Work out the finished part from the listing and answer in its coordinate system (mm). Face numbers are marked on the shaded views. A direction names the side the tool comes from. Round coordinates to 2 decimals unless told otherwise and drop trailing zeros. Order: outer loops, then holes, each group sorted by start corner. A loop starts at its lowest first (then second) coordinate and runs counter-clockwise, first axis right, second up. Notation, with made-up numbers: (-3, 67.5) - (52, 67.5) arc R26 cw to (52, 106.5) - close; hole circle Ø5 at (-19, 2). An arc over 180 degrees is marked (long way). Answer in a Markdown table with one row per item.
from build123d import *

# Parameters (mm, degrees)
ESQUISSE2_W           = 165
ESQUISSE2_H           = 165
BASE_DEPTH            = 30
ESQUISSE3_R           = 15
BLOC_MOTEUR_1_DEPTH   = 80
ESQUISSE4_W           = 10
ESQUISSE4_H           = 22.360679774
ACCES_MOTEUR_DEPTH    = 37
ESQUISSE6_R           = 16.01
BLOC_MOTEUR_2_DEPTH   = 37
ESQUISSE7_R           = 2.5
VIS_MOTEUR_DEPTH      = 121.467838032
ESQUISSE8_R           = 2.5
VIS_PATIN_DEPTH       = 121.467838032
ESQUISSE9_R           = 3.1
ESQUISSE9_R_2         = 1.375
SUPPORT_RASP_DEPTH    = 10
ESQUISSE11_R          = 2.5
ESQUISSE11_R_2        = 1.6
SUPPORT_ARDUINO_DEPTH = 10
CONGE_EXT_R           = 5
ESQUISSE12_R          = 30
ESPACE_ROUE_DEPTH     = 10


with BuildPart() as part:
    # Esquisse2 → BASE (new body)
    with BuildSketch(Plane(origin=(0, 0, 0), x_dir=(1, 0, 0), z_dir=(0, 1, 0))):
        Rectangle(ESQUISSE2_W, ESQUISSE2_H)
    extrude(amount=BASE_DEPTH)

    # Esquisse3 → BLOC MOTEUR 1. (cut)
    with BuildSketch(Plane(origin=(82.5, 0, 0), x_dir=(0, 0, -1), z_dir=(1, 0, 0))):
        with Locations((50, 10)):
            Circle(ESQUISSE3_R)
    bloc_moteur_1 = extrude(amount=-BLOC_MOTEUR_1_DEPTH, mode=Mode.SUBTRACT)

    # Esquisse4 → ACCES MOTEUR (cut)
    with BuildSketch(Plane.XZ):
        with Locations((7.5, -50)):
            Rectangle(ESQUISSE4_W, ESQUISSE4_H)
    acces_moteur = extrude(amount=-ACCES_MOTEUR_DEPTH, mode=Mode.SUBTRACT)

    # Esquisse6 → BLOC MOTEUR 2 (cut)
    with BuildSketch(Plane(origin=(82.5, 0, 0), x_dir=(0, 0, -1), z_dir=(1, 0, 0))):
        with Locations((50, 10)):
            Circle(ESQUISSE6_R)
    bloc_moteur_2 = extrude(amount=-BLOC_MOTEUR_2_DEPTH, mode=Mode.SUBTRACT)

    # SYM BLOC MOTEUR: BLOC MOTEUR 1., ACCES MOTEUR, BLOC MOTEUR 2 across plane
    add(bloc_moteur_1.mirror(Plane(origin=(0, 0, 0), x_dir=(0, 0, 1), z_dir=(1, 0, 0))), mode=Mode.SUBTRACT)
    add(acces_moteur.mirror(Plane(origin=(0, 0, 0), x_dir=(0, 0, 1), z_dir=(1, 0, 0))), mode=Mode.SUBTRACT)
    add(bloc_moteur_2.mirror(Plane(origin=(0, 0, 0), x_dir=(0, 0, 1), z_dir=(1, 0, 0))), mode=Mode.SUBTRACT)

    # Esquisse7 → VIS MOTEUR (cut, through all)
    with BuildSketch(Plane.XZ):
        with Locations(Location((-64, -27.497196314, 0), (0, 0, 270))):
            Circle(ESQUISSE7_R)
        with Locations(Location((-24, -28.819660113, 0), (0, 0, 270))):
            Circle(ESQUISSE7_R)
        with Locations(Location((-24, -71.180339887, 0), (0, 0, 270))):
            Circle(ESQUISSE7_R)
        with Locations(Location((-64, -72.502803686, 0), (0, 0, 270))):
            Circle(ESQUISSE7_R)
    vis_moteur = extrude(amount=-VIS_MOTEUR_DEPTH, mode=Mode.SUBTRACT)

    # SYM VIS: VIS MOTEUR across plane
    add(vis_moteur.mirror(Plane(origin=(0, 0, 0), x_dir=(0, 0, 1), z_dir=(1, 0, 0))), mode=Mode.SUBTRACT)

    # Esquisse8 → VIS PATIN (cut, through all)
    with BuildSketch(Plane.XZ):
        with Locations(Location((-52.5, 52.5, 0), (0, 0, 270))):
            Circle(ESQUISSE8_R)
        with Locations(Location((52.5, 52.5, 0), (0, 0, 270))):
            Circle(ESQUISSE8_R)
    extrude(amount=-VIS_PATIN_DEPTH, mode=Mode.SUBTRACT)

    # Esquisse9 → SUPPORT RASP (add)
    # profile 1 of 4: a face of its own
    with BuildSketch(Plane(origin=(0, 30, 0), x_dir=(1, 0, 0), z_dir=(0, 1, 0))):
        with Locations(Location((-5.124679211, -22.194338496, 0), (0, 0, 90))):
            Circle(ESQUISSE9_R)
        with Locations(Location((-5.124679211, -22.194338496, 0), (0, 0, 270))):
            Circle(ESQUISSE9_R_2, mode=Mode.SUBTRACT)
    # profile 2 of 4: a face of its own
    with BuildSketch(Plane(origin=(0, 30, 0), x_dir=(1, 0, 0), z_dir=(0, 1, 0))):
        with Locations(Location((52.875320789, -22.194338496, 0), (0, 0, 90))):
            Circle(ESQUISSE9_R)
        with Locations(Location((52.875320789, -22.194338496, 0), (0, 0, 270))):
            Circle(ESQUISSE9_R_2, mode=Mode.SUBTRACT)
    # profile 3 of 4: a face of its own
    with BuildSketch(Plane(origin=(0, 30, 0), x_dir=(1, 0, 0), z_dir=(0, 1, 0))):
        with Locations(Location((-5.124679211, -71.194338496, 0), (0, 0, 90))):
            Circle(ESQUISSE9_R)
        with Locations(Location((-5.124679211, -71.194338496, 0), (0, 0, 270))):
            Circle(ESQUISSE9_R_2, mode=Mode.SUBTRACT)
    # profile 4 of 4: a face of its own
    with BuildSketch(Plane(origin=(0, 30, 0), x_dir=(1, 0, 0), z_dir=(0, 1, 0))):
        with Locations(Location((52.875320789, -71.194338496, 0), (0, 0, 90))):
            Circle(ESQUISSE9_R)
        with Locations(Location((52.875320789, -71.194338496, 0), (0, 0, 270))):
            Circle(ESQUISSE9_R_2, mode=Mode.SUBTRACT)
    extrude(amount=SUPPORT_RASP_DEPTH)

    # Esquisse11 → SUPPORT ARDUINO (add)
    # profile 1 of 4: a face of its own
    with BuildSketch(Plane(origin=(0, 30, 0), x_dir=(1, 0, 0), z_dir=(0, 1, 0))):
        with Locations(Location((-70.933772323, -17.670594659, 0), (0, 0, 90))):
            Circle(ESQUISSE11_R)
        with Locations(Location((-70.933772323, -17.670594659, 0), (0, 0, 270))):
            Circle(ESQUISSE11_R_2, mode=Mode.SUBTRACT)
    # profile 2 of 4: a face of its own
    with BuildSketch(Plane(origin=(0, 30, 0), x_dir=(1, 0, 0), z_dir=(0, 1, 0))):
        with Locations(Location((-23.123772323, -18.770594659, 0), (0, 0, 90))):
            Circle(ESQUISSE11_R)
        with Locations(Location((-23.123772323, -18.770594659, 0), (0, 0, 270))):
            Circle(ESQUISSE11_R_2, mode=Mode.SUBTRACT)
    # profile 3 of 4: a face of its own
    with BuildSketch(Plane(origin=(0, 30, 0), x_dir=(1, 0, 0), z_dir=(0, 1, 0))):
        with Locations(Location((-66.233772323, -60.010594659, 0), (0, 0, 90))):
            Circle(ESQUISSE11_R)
        with Locations(Location((-66.233772323, -60.010594659, 0), (0, 0, 270))):
            Circle(ESQUISSE11_R_2, mode=Mode.SUBTRACT)
    # profile 4 of 4: a face of its own
    with BuildSketch(Plane(origin=(0, 30, 0), x_dir=(1, 0, 0), z_dir=(0, 1, 0))):
        with Locations(Location((-38.333772323, -60.010594659, 0), (0, 0, 90))):
            Circle(ESQUISSE11_R)
        with Locations(Location((-38.333772323, -60.010594659, 0), (0, 0, 270))):
            Circle(ESQUISSE11_R_2, mode=Mode.SUBTRACT)
    extrude(amount=SUPPORT_ARDUINO_DEPTH)

    # CONGE EXT
    conge_ext_edges = [part.edges().sort_by_distance(p)[0] for p in [
        (-82.5, 15, -82.5),
        (82.5, 15, -82.5),
        (82.5, 15, 82.5),
        (-82.5, 15, 82.5),
    ]]
    fillet(conge_ext_edges, radius=CONGE_EXT_R)

    # Esquisse12 → ESPACE ROUE (cut)
    with BuildSketch(Plane.ZY.offset(82.5)):
        with Locations((-50, 10)):
            Circle(ESQUISSE12_R)
    espace_roue = extrude(amount=-ESPACE_ROUE_DEPTH, mode=Mode.SUBTRACT)

    # SYM ESPACE ROUE: ESPACE ROUE across plane
    add(espace_roue.mirror(Plane(origin=(0, 0, 0), x_dir=(0, 0, 1), z_dir=(1, 0, 0))), mode=Mode.SUBTRACT)


solid = part.part
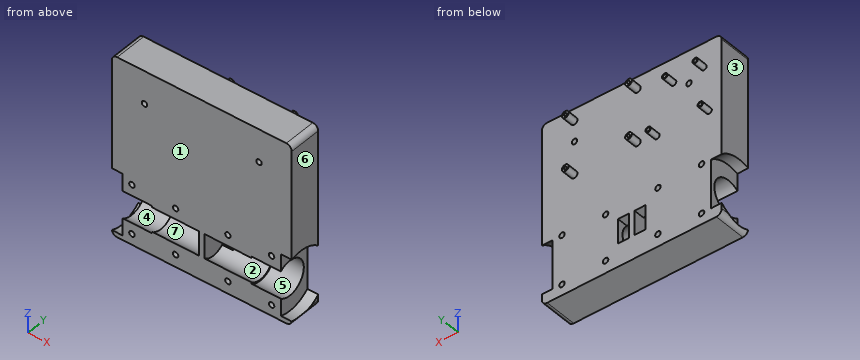
1) Find section B-B, the plane x = 24. Give the vertices of the cut face in (y, z), then the cut area to 3 significant figures.
Filled in:
| item | result |
|---|---|
| outline | (0, -82.5) - (30, -82.5) - (30, -73.68) - (0, -73.68) - close; (0, -68.68) - (30, -68.68) - (30, -31.32) - (0, -31.32) - (0, -38.82) arc R15 cw (long way) to (0, -61.18) - close; (0, -26.32) - (30, -26.32) - (30, 82.5) - (0, 82.5) - close |
| area | 4,020 mm^2 |
2) Find section D-D, the plane y = 16. Give the number of separate pieces and of enclosed holes in the cut face, then the cut area to 3 significant figures.
Filled in:
| item | result |
|---|---|
| separate pieces | 1 |
| enclosed holes | 10 |
| area | 21,900 mm^2 |
3) Find section C-C, the plane x = -52.5. Give the vertices of the cut face in (y, z).
Filled in:
| item | result |
|---|---|
| outline | (0, -82.5) - (30, -82.5) - (30, 50) - (0, 50) - (0, -37.5) arc R16.01 cw (long way) to (0, -62.5) - close; (0, 55) - (30, 55) - (30, 82.5) - (0, 82.5) - close |
4) Find section A-A, the plane z = 52.5. Give the vertices of the cut face in (x, y).
Filled in:
| item | result |
|---|---|
| outline | (-82.5, 0) - (-55, 0) - (-55, 30) - (-82.5, 30) - close; (-50, 0) - (50, 0) - (50, 30) - (-50, 30) - close; (55, 0) - (82.5, 0) - (82.5, 30) - (55, 30) - close |
5) Each of these flat-tipped pins is pushed along its axis until it touches: pin 1 (1.5 mm diameter, centred on y = 31, z = 42.5, fed in from +X); pin 2 (1.6 mm diameter, centred on x = -66.5, z = 60.5, fed in from +Y); pin 3 (24 mm diameter, centred on y = 19.5, z = -51.5, fed in from -X); pin 4 (24 mm diameter, centred on y = 20.5, z = -48, fed in from +X). Where does it stop, or does it pass through?
Filled in:
| item | result |
|---|---|
| pin 1 | passes through |
| pin 2 | stops at y = 30 |
| pin 3 | stops at x = -72.5 |
| pin 4 | stops at x = 72.5 |
6) Which of the six approach directions +Z, -Z, +X, -X, +Y, -Y give full straight-line access (tool end or side, diameter ignored) to the marked faces 5, 6 and 7?
Filled in:
| item | result |
|---|---|
| face 5 | +X |
| face 6 | +Z, -Z, +X, +Y, -Y |
| face 7 | -X |
7) Find the intervals of material crossed by probe 1 along Z at (x, y) = (61, 10); probe 2 along Z at (x, y) = (-43.5, 11); probe 3 along Z at (x, y) = (52, 37.5), in increasing order. Write a range as from..to.
Filled in:
| item | result |
|---|---|
| probe 1 | z = -82.5..-66.01, -33.99..82.5 |
| probe 2 | z = -82.5..-64.97, -35.03..82.5 |
| probe 3 | z = 19.22..21.13, 23.25..25.17, 68.22..70.13, 72.25..74.17 |
8) The mould has two halves that part along Y. Classify the marked faces 1, 2, 3 and 4: released by +Y, released by -Y, zero draft, split by the parting line, or undercut.
Filled in:
| item | result |
|---|---|
| face 1 | released by -Y |
| face 2 | undercut |
| face 3 | zero draft |
| face 4 | undercut |
